Could you check a few things on this drawing? It's one solid part, dimensions in mm from its lowest x, y, z. A direction names the side the tool comes from. Coordinates: 2 decimals unless noted, no trailing zeros. Order: outer loops, then holes, each group sorted by start corner. A loop starts at its lowest first (then second) coordinate and runs counter-clockwise, first axis right, second up. Notation, with made-up numbers: (-25, 14) -> (-4, 14) arc R11 ccw to (-4, 22) -> close; hole circle Ø10 at (-10.75, 17.5). An arc over 180 degrees is marked (long way). Answer as CSV lines item,"result".
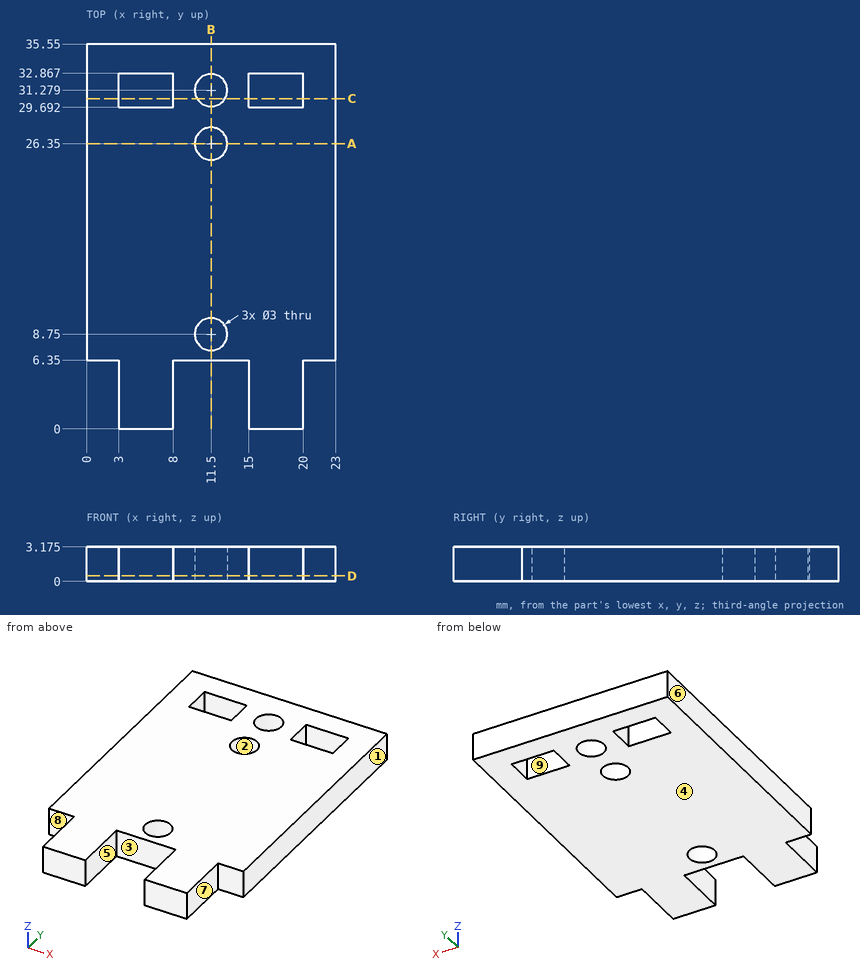
Q1. Imagine slicing it at A-A (y = 26.35). List the corners of the cut face in (x, z) for me (1 decimal), and give its area (3 significant figures).
Solution:
outline,"(0, 0) -> (10, 0) -> (10, 3.2) -> (0, 3.2) -> close; (13, 0) -> (23, 0) -> (23, 3.2) -> (13, 3.2) -> close"
area,"63.5 mm2"
Q2. If I drill on line 1 (Y direction, x = 11.5, z = 1.4); line 2 (X direction, y = 26.35, z = 0.75); line 3 (Y direction, x = 19, z = 1.6), over which ranges is the centre line in solid material (lowest first)?
Solution:
line 1,"6.35 to 7.25, 10.25 to 24.85, 27.85 to 29.78, 32.78 to 35.55"
line 2,"0 to 10, 13 to 23"
line 3,"0 to 29.69, 32.87 to 35.55"
Q3. Imagine slicing it at B-B (x = 11.5). Give the number of separate pieces and of enclosed holes in the cut face.
Solution:
separate pieces,"4"
enclosed holes,"0"
Q4. Imagine slicing it at C-C (y = 30.5). List the corners of the cut face in (x, z) for me (1 decimal).
Solution:
outline,"(0, 0) -> (3, 0) -> (3, 3.2) -> (0, 3.2) -> close; (8, 0) -> (10.2, 0) -> (10.2, 3.2) -> (8, 3.2) -> close; (12.8, 0) -> (15, 0) -> (15, 3.2) -> (12.8, 3.2) -> close; (20, 0) -> (23, 0) -> (23, 3.2) -> (20, 3.2) -> close"
Q5. Imagine slicing it at D-D (z = 0.5). List the corners of the cut face in (x, y) for me, and give its area (3 significant figures).
Solution:
outline,"(0, 6.35) -> (3, 6.35) -> (3, 0) -> (8, 0) -> (8, 6.35) -> (15, 6.35) -> (15, 0) -> (20, 0) -> (20, 6.35) -> (23, 6.35) -> (23, 35.55) -> (0, 35.55) -> close; hole (3, 29.69) -> (8, 29.69) -> (8, 32.87) -> (3, 32.87) -> close; hole circle Ø3 at (11.5, 8.75); hole circle Ø3 at (11.5, 26.35); hole circle Ø3 at (11.5, 31.28); hole (15, 29.69) -> (20, 29.69) -> (20, 32.87) -> (15, 32.87) -> close"
area,"682 mm2"
Q6. For P1, Ø2.5, axis at x = 11.5, y = 31.28, coming from the +Z side; P2, Ø1.6, axis at y = 3, z = 2, coming from the -X side; P3, Ø1.6, axis at y = 3.5, z = 2, coming from the +X side, each with a flat end and sliding along its axis, tell me the tip position at first contact or that it passes through.
Solution:
P1,"through"
P2,"x = 3"
P3,"x = 20"
Q7. Which directions (+Z, -Z, +X, -X, +Y, -Y) give clear straight access to the entire face, cutting with the end or side of a thin tool? Please do the marked faces 5, 6, 7, 8 and 9.
Solution:
face 5,"+Z, -Z, -Y"
face 6,"+Z, -Z, -X, +Y, -Y"
face 7,"+Z, -Z, +X, -Y"
face 8,"+Z, -Z, -X, -Y"
face 9,"+Z, -Z"
Q8. We'd pull the mould along X, two halves only. Please class the marked faces 1, 2, 3 and 4: pulls with the +X half, pulls with the -X half, needs draft (parallel to the pull), parting line crosses it, or undercut.
Solution:
face 1,"pulls with the +X half"
face 2,"undercut"
face 3,"undercut"
face 4,"needs draft"
